Source: CAD feature listing. Evaluate the final solid. Frame: model axes, mm. Face numbers are marked on the shaded views. A direction names the side the tool comes from. Coordinates: 2 decimals unless noted, no trailing zeros. Write each loop counter-clockwise with the first axis right and the second up, starting at its lowest first coordinate (ties: lowest second). Pieces come first, ordered by that corner, then holes. Notation, with made-up numbers: M 9.25,1.25 L 35.25,1.25 A13 ccw 35.25,18.25 Z; hole C 71.25,-4.75 d11. An arc over 180 degrees is marked long. Write item = value, one per line. Start each with the question number.
1. Line query: line 1 along Y through (x, z) = (0, -3.25); line 2 along Z through (x, y) = (3, -2); line 3 along Z through (x, y) = (1.25, 3.75). Output: solid intervals per line, ascending.
2. Pin query (flat end, axial travel): pin 1 Ø6 at (x, z) = (3.5, -23) entering from +Y; pin 2 Ø4 at (x, z) = (2, -9) entering from +Y; pin 3 Ø6 at (x, z) = (1.5, -20.5) entering from -Y. Return the tip coordinate at first contact, or that it passes through.
3. Section query C-C (z = -26.5). Output: boundary loops of the cut face in (x, y), then the cut area to 3 significant figures.
4. Section query A-A (z = -6). Output: boundary loops of the cut face in (x, y), then the cut area to 3 significant figures.
5. Access query for the marked faces 1 and 2. Directions: +Z, -Z, +X, -X, +Y, -Y. A direction counts if a zero-diameter tool reaches every point of the face in a straight line with its end or side. Return the directions, or none.
6. Pull-direction query (Y, two-part tool) for the marked faces 3, 4 and 5; classes: pulls with the +Y half, pulls with the -Y half, needs draft (parallel to the pull), parting line crosses it, or undercut.
7. Section query B-B (z = -9.5). Output: boundary loops of the cut face in (x, y), then the cut area to 3 significant figures.
Autodesk Inventor part; units mm, degrees
ref_plane "MSC_PF1" through (0, 0, 0) normal (0, 1, 0) x (-1, 0, 0)
ref_plane "MSC_PT1" through (0, 0, -6.6669) normal (0, 0, -1) x (-1, 0, 0)
ref_plane "YZ Plane" through (0, 0, 0) normal (1, 0, 0) x (0, 1, 0)
sketch "Sketch2" plane through (0, 0, 0) normal (0, 1, 0) x (-1, 0, 0)
  line L0 (0, -6.6669) -> (0, -36.6669)
  line L1 (0, -36.6669) -> (2.5, -36.6669)
  line L2 (3, -36.1669) -> (3, -18.6669)
  line L3 (3, -18.6669) -> (2.65, -18.0607)
  line L4 (2.65, -18.0607) -> (2.65, -6.6669)
  line L5 (2.65, -6.6669) -> (0, -6.6669)
  line L6 (2.5, -36.6669) -> (3, -36.1669)
  line L7 (3, -36.6669) -> (3, -37.374)
  line L8 (0, -43.5155) -> (0, -0.5255)
  dimension "Ds" = 5.3
  dimension "NND" = 6
  dimension "b" = 18
  dimension "d3" = 30
  dimension "d5" = 45
  dimension "PTC" = 1
  dimension "NLG" = 30
revolve "Revolution1" add sketch "Sketch2" angle 360 about axis through (0, 0, -6.6669) along (0, 0, -1)
sketch "Sketch3" plane through (0, 0, -6.6669) normal (0, 0, 1) x (1, 0, 0)
  circle A0 centre (0, 0) radius 2.65
  line L0 (0, 5) -> (2.8868, 5)
  line L1 (2.8868, 5) -> (5.7735, 0)
  line L2 (5.7735, 0) -> (0, 0)
  line L3 (0, 0) -> (0, 5)
  line L4 (0, 5) -> (-2.8868, 5)
  line L5 (-2.8868, 5) -> (-5.7735, 0)
  line L6 (0, -5) -> (2.8868, -5)
  line L7 (2.8868, -5) -> (5.7735, 0)
  line L8 (-2.8868, -5) -> (-5.7735, 0)
  line L9 (0, -5) -> (-2.8868, -5)
  dimension "d9" = 60
  dimension "ParS" = 10
  dimension "msp_d11" = 10
extrude "Extrusion1" add sketch "Sketch3" along normal blind 4
sketch "Sketch4" plane through (0, 0, 0) normal (0, 1, 0) x (-1, 0, 0)
  line L0 (-5, -2.6669) -> (-5.7735, -2.6669)
  line L1 (-5.7735, -2.6669) -> (-5.7735, -3.1135)
  line L2 (-5.7735, -3.1135) -> (-5, -2.6669)
  line L3 (0, -13.5254) -> (0, 34.4838)
  line L4 (0, 27.6253) -> (0, 27.1787)
  line L5 (-5.7735, -6.6669) -> (-5.7735, -2.6669)
  line L6 (-2.8868, -2.6669) -> (-5.7735, -2.6669)
  dimension "d14" = 30
  dimension "msp_d15" = 10
revolve "Revolution2" cut sketch "Sketch4" angle 360 about axis through (0, 0, 27.6253) along (0, 0, -1)
sketch "Sketch5" plane through (0, 0, -2.6669) normal (0, 0, 1) x (1, 0, 0)
  arc A0 (4.3301, 2.5) -> (0, 5) centre (0, 0) ccw
  circle A1 centre (0, 0) radius 3.75
  dimension "d27" = 7.5
extrude "Extrusion2" cut sketch "Sketch5" against normal blind 0.8
thread "Thread1"
ref_plane "MSC_PF1" through (0, 0, 0) normal (0, 1, 0) x (-1, 0, 0)
ref_plane "MSC_PT1" through (0, 0, -6.6669) normal (0, 0, -1) x (-1, 0, 0)
fillet "Fillet1" radius 0.25 1 edges at (2.65, 0, -6.6669)
equation "\"msp_d11\" = ParS"
equation "\"msp_d15\" = ParS"
equation "\"d27\" = 0.75 * ParS"
equation "\"d28\" = 0.2 * ParK"
equation "\"d30\" = r"
equation "\"msp_d17\" = b"
equation "\"r\" = 0.25"
equation "\"THREADDIA\" = NND"
properties part number "ISO 4015 - M6 x 30" material "Stainless Steel, 440C"
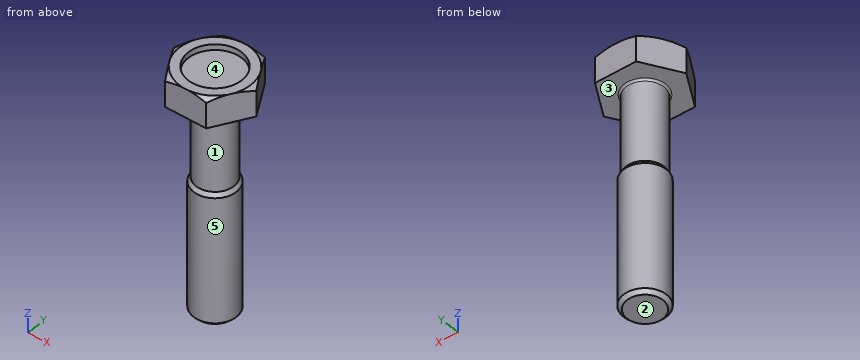
Results are:
q1.line_1 = -5 to -3.75, 3.75 to 5
q1.line_2 = -6.67 to -3.47
q1.line_3 = -6.67 to -2.67
q2.pin_1 = 2.96
q2.pin_2 = 2.65
q2.pin_3 = -3
q3.outline = C 0,0 d6
q3.area = 28.3 mm^2
q4.outline = M -5.77,0 L -2.89,-5 L 2.89,-5 L 5.77,0 L 2.89,5 L -2.89,5 Z
q4.area = 86.6 mm^2
q5.face_1 = none
q5.face_2 = -Z, +X, -X, +Y, -Y
q6.face_3 = needs draft
q6.face_4 = undercut
q6.face_5 = parting line crosses it
q7.outline = C 0,0 d5.3
q7.area = 22.1 mm^2
